Could you check a few things on this drawing? It's one solid part, dimensions in mm from its lowest x, y, z. Round coordinates to 2 decimals unless told otherwise and drop trailing zeros. Write each loop counter-clockwise with the first axis right and the second up, starting at its lowest first coordinate (ties: lowest second). Pieces come first, ordered by that corner, then holes. Notation, with made-up numbers: (72, 43) -> (126, 43) arc R14 ccw to (126, 57) -> close; hole circle Ø4 at (19.25, -22.75). An arc over 180 degrees is marked (long way). Answer in a Markdown table with one row per item.
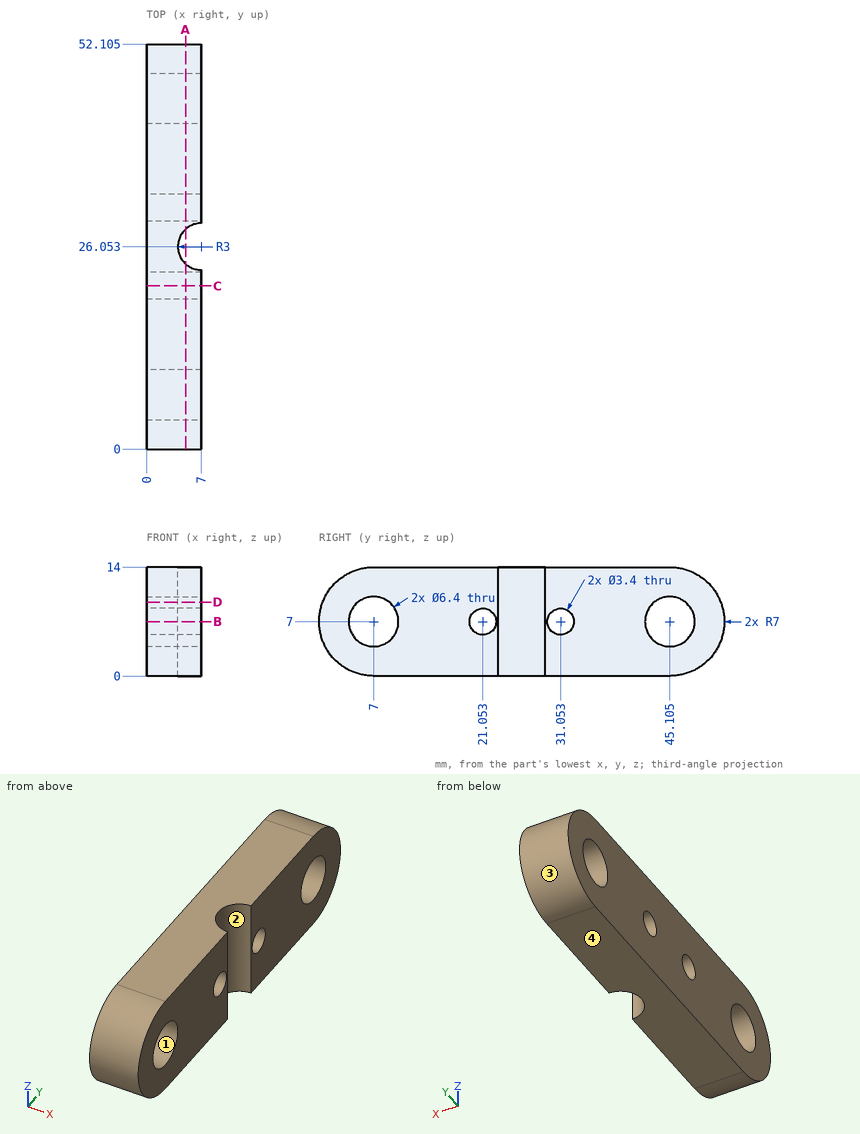
1) For pin 1 (3 mm diameter, centred on y = 21.05, z = 7, fed in from -X); pin 2 (3 mm diameter, centred on x = 4, z = 2.5, fed in from +Y); pin 3 (2 mm diameter, centred on x = 2, z = 12, fed in from +Y), each with a flat end and sliding along its axis, tell me the tip position at first contact or that it passes through.
Findings:
| item | result |
|---|---|
| pin 1 | passes through |
| pin 2 | stops at y = 51.43 |
| pin 3 | stops at y = 50.85 |
2) Imagine slicing it at C-C, the plane y = 21. Please give me the cut outline in (x, z).
Findings:
| item | result |
|---|---|
| outline | (0, 0) -> (7, 0) -> (7, 5.3) -> (0, 5.3) -> close; (0, 8.7) -> (7, 8.7) -> (7, 14) -> (0, 14) -> close |
3) Imagine slicing it at D-D, the plane z = 9.5. Please give me the cut outline in (x, y), plus the area to 3 significant figures.
Findings:
| item | result |
|---|---|
| outline | (0, 0.46) -> (7, 0.46) -> (7, 5) -> (0, 5) -> close; (0, 9) -> (7, 9) -> (7, 23.05) arc R3 cw to (7, 29.05) -> (7, 43.11) -> (0, 43.11) -> close; (0, 47.1) -> (7, 47.1) -> (7, 51.64) -> (0, 51.64) -> close |
| area | 288 mm^2 |
4) Imagine slicing it at B-B, the plane z = 7. Count the separate pieces of the cut face and the enclosed holes in it.
Findings:
| item | result |
|---|---|
| separate pieces | 5 |
| enclosed holes | 0 |
5) Please list where these lines run through material, in increasing order: line 1 (Y direction, x = 3, z = 6.5) (1 decimal); line 2 (Z direction, x = 4.75, y = 7); line 3 (Y direction, x = 4.5, z = 6.5) (1 decimal).
Findings:
| item | result |
|---|---|
| line 1 | y = 0 to 3.8, 10.2 to 19.4, 22.7 to 29.4, 32.7 to 41.9, 48.3 to 52.1 |
| line 2 | z = 0 to 3.8, 10.2 to 14 |
| line 3 | y = 0 to 3.8, 10.2 to 19.4, 22.7 to 24.4, 27.7 to 29.4, 32.7 to 41.9, 48.3 to 52.1 |
6) Imagine slicing it at A-A, the plane x = 5. Please give me the cut outline in (y, z) (1 decimal), plus the area to 3 significant figures.
Findings:
| item | result |
|---|---|
| outline | (7, 0) -> (23.8, 0) -> (23.8, 14) -> (7, 14) arc R7 ccw to start; (28.3, 0) -> (45.1, 0) arc R7 ccw to (45.1, 14) -> (28.3, 14) -> close; hole circle Ø6.4 at (7, 7); hole circle Ø3.4 at (21.1, 7); hole circle Ø3.4 at (31.1, 7); hole circle Ø6.4 at (45.1, 7) |
| area | 542 mm^2 |
7) Thinking about a two-plate mould opening in Y: for the marked faces 1, 2, 3 and 4, which applies, +Y half, -Y half, draft (parallel to the pull), parting line (faces both ways), or undercut?
Findings:
| item | result |
|---|---|
| face 1 | undercut |
| face 2 | undercut |
| face 3 | +Y half |
| face 4 | draft |
